Verification items for the finished model (mm, model axes). A direction names the side the tool comes from. Round coordinates to 2 decimals unless told otherwise and drop trailing zeros. Order: outer loops, then holes, each group sorted by start corner. A loop starts at its lowest first (then second) coordinate and runs counter-clockwise, first axis right, second up. Notation, with made-up numbers: M 48.25,70.5 L 67.25,70.5 A14 ccw 67.25,76.5 Z; hole C 34.25,13 d3. An arc over 180 degrees is marked long. Answer as a JSON object with one key per item and string values. Group by question number.
```python
from build123d import *

# Parameters (mm, degrees)
F1_DEPTH = 150
F3_ANGLE = 90
F4_DEPTH = 50


with BuildPart() as f1:
    # F0 (on Front) → F1 (new body)
    with BuildSketch(Plane.XZ):
        Polygon((22.9738393507, -9.6457333625), (28.5607396108, -0.0310617447), (23.0276398708, 9.6146716177), (11.9076398708, 9.6457333625), (6.3207396108, 0.0310617447), (11.8538393507, -9.6146716177), align=None)
    extrude(amount=F1_DEPTH)

    # F2 (on face) → F3 (revolve)
    with BuildSketch(Plane.XZ.offset(150)):
        Polygon((11.9076398708, 9.6457333625), (6.3207396108, 0.0310617447), (11.8538393507, -9.6146716177), (22.9738393507, -9.6457333625), (28.5607396108, -0.0310617447), (23.0276398708, 9.6146716177), align=None)
    revolve(axis=Axis((6.3207396108, -150, 14.933847028), (0, 0, -1)), revolution_arc=F3_ANGLE)

    # F4 (add): a face of the model
    f4_faces = [f1.faces().sort_by_distance(p)[0] for p in [
        (6.3207396108, -161.12, 0),
    ]]
    extrude(f4_faces, amount=F4_DEPTH)


solid = f1.part
```
Q1. Thickness scan on line 1 (Z direction, x = 11, y = -162.5); line 2 (Y direction, x = -30, z = 7.75); line 3 (X direction, y = -17, z = 0.25). Record the ranges inside material, lowest first. Write a range as from..to.
Q2. Cross-section at D-D, the plane z = 6.5. Record the cut outline in (x, y), then the cut area to 3 significant figures.
Q3. Tool access check on faces 1 (the face through (9.049, -73.95, -4.724)), 2 (the face through (19.774, -163.161, 5.931)), 3 (the face through (-18.329, -152.833, 4.906)). Record the directions out of +Z, -Z, +X, -X, +Y, -Y that give a thin tool (end or side, any length) a straight path to the whole face; none if there is none.
Q4. Cross-section at B-B, the plane z = -8. Record the cut outline in (x, y), then the cut area to 3 significant figures.
Q5. Cross-section at A-A, the plane y = -31. Record the cut outline in (x, z).
Q6. Gauge pin test, flat ends, axial feed: pin 1 Ø2 at (x, z) = (-14, 2) entering from -Y; pin 2 Ø2 at (x, y) = (4.5, -138) entering from +Z; pin 3 Ø10 at (x, y) = (2.5, -73.5) entering from +Z; pin 4 Ø2 at (x, z) = (-32.5, -3) entering from -Y. Record the tip position at first contact, or that the pin passes through.
Q7. Cross-section at C-C, the plane x = -13.5. Record the cut outline in (y, z).
Conclusion:
{
 "1": {"line 1": "-9.64..9.62", "line 2": "-167.78..-154.49", "line 3": "6.45..28.4"},
 "2": {"outline": "M -43.68,-168.49 L 6.32,-168.49 A18.49 ccw 24.81,-150 L 24.81,0 L 10.08,0 L 10.08,-150 A3.76 cw 6.32,-153.76 L -43.68,-153.76 Z", "area": "3,200 mm2"},
 "3": {"face 1": "-Z, -X, +Y", "face 2": "+Z, +X, -Y", "face 3": "+Z, -X, +Y"},
 "4": {"outline": "M -43.68,-167.61 L 6.32,-167.61 A17.61 ccw 23.93,-150 L 23.93,0 L 10.93,0 L 10.93,-150 A4.61 cw 6.32,-154.61 L -43.68,-154.61 Z", "area": "2,830 mm2"},
 "5": {"outline": "M 6.32,0.03 L 11.85,-9.61 L 22.97,-9.65 L 28.56,-0.03 L 23.03,9.61 L 11.91,9.65 Z"},
 "6": {"pin 1": "y = -171.65", "pin 2": "through", "pin 3": "z = 2.06", "pin 4": "y = -171.1"},
 "7": {"outline": "M -172.24,-0.03 L -166.65,-9.65 L -155.53,-9.61 L -150,0.03 L -155.59,9.65 L -166.71,9.61 Z"}
}
